```python
from build123d import *

# Parameters (mm, degrees)
BOSS_EXTRUDE1_DEPTH = 1.25
BOSS_EXTRUDE4_START = -15.5
SKETCH1_5_R         = 2
BOSS_EXTRUDE4_DEPTH = 16.75
SKETCH1_6_R         = 2
BOSS_EXTRUDE5_DEPTH = 30
CIRPATTERN1_COUNT   = 3


with BuildPart() as part:
    # Sketch1 → Boss-Extrude1 (new body, symmetric)
    with BuildSketch(Plane.XY):
        with BuildLine():
            Line((50, 2), (0, 2))
            ThreePointArc((0, 2), (1.414213562, 1.414213562), (2, 0))
            ThreePointArc((2, 0), (1.414213562, -1.414213562), (0, -2))
            Line((0, -2), (50, -2))
            ThreePointArc((50, -2), (48, 0), (50, 2))
        make_face()
    boss_extrude1 = extrude(amount=BOSS_EXTRUDE1_DEPTH, both=True)

    # Sketch1_5 → Boss-Extrude4 (add)
    with BuildSketch(Plane.XY.offset(BOSS_EXTRUDE4_START)):
        Circle(SKETCH1_5_R)
        with Locations((50, 0)):
            Circle(SKETCH1_5_R)
    boss_extrude4 = extrude(amount=BOSS_EXTRUDE4_DEPTH)

    # Sketch1_6 → Boss-Extrude5 (add)
    with BuildSketch(Plane.XY):
        Circle(SKETCH1_6_R)
    extrude(amount=BOSS_EXTRUDE5_DEPTH)

    # CirPattern1: Boss-Extrude1, Boss-Extrude4 ×3 about axis
    cirpattern1_axis = Axis((0, 0, 0), (0, 0, 1))
    for i in range(1, CIRPATTERN1_COUNT):
        add(boss_extrude1.rotate(cirpattern1_axis, i * 360 / CIRPATTERN1_COUNT))
        add(boss_extrude4.rotate(cirpattern1_axis, i * 360 / CIRPATTERN1_COUNT))


solid = part.part
```
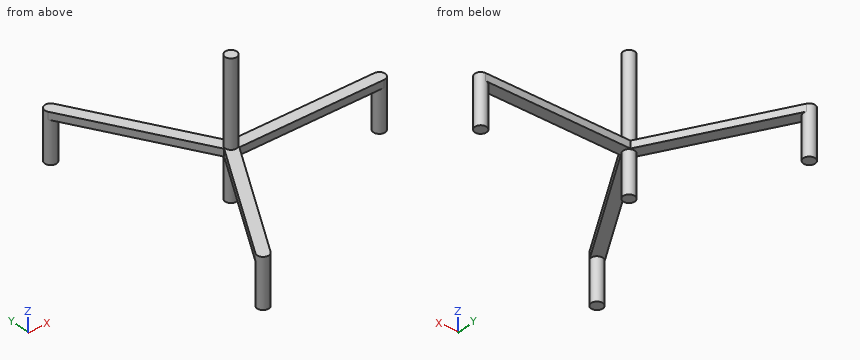
Part model, mm, in its own coordinate system. Round coordinates to 2 decimals unless told otherwise and drop trailing zeros. Order: outer loops, then holes, each group sorted by start corner. A loop starts at its lowest first (then second) coordinate and runs counter-clockwise, first axis right, second up. Notation, with made-up numbers: M -40,75 L -14,75 A31 cw -14,101 Z; hole C -1,23 d9. An arc over 180 degrees is marked long. Put each result on its own line as item: value. Start each with the question number.
1. Drill centre lines: probe 1 along Z at (x, y) = (-23.5, -37); probe 2 along Y at (x, z) = (8.5, -1); probe 3 along Y at (x, z) = (-1, 16). Where is each one in solid material? Low to high. Write a range as [from, to].
2. Drop flat-ended pins along their axis: pin 1 (12 mm diameter, centred on y = -15.5, z = 0, fed in from -X); pin 2 (3 mm diameter, centred on y = -3, z = 23, fed in from -X); pin 3 (3 mm diameter, centred on x = 26, z = 0, fed in from -Y). Give the stop position or say it passes through.
3. Slice it at C-C on z = -3. List the corners of the cut face in (x, y).
4. Slice it at A-A on z = 5.5. List the corners of the cut face in (x, y).
5. Slice it at D-D on y = -4. List the corners of the cut face in (x, z).
6. Slice it at B-B on x = 15. List the corners of the cut face in (y, z).
Findings:
1. probe 1: [-1.25, 1.25]
1. probe 2: [-2, 2]
1. probe 3: [-1.73, 1.73]
2. pin 1: x = -14.72
2. pin 2: x = -1.32
2. pin 3: y = -2
3. outline: C -25,-43.3 d4; C -25,43.3 d4; C 0,0 d4; C 50,0 d4
4. outline: C 0,0 d4
5. outline: M -4.62,-1.25 L 0,-1.25 L 0,1.25 L -4.62,1.25 Z
6. outline: M -2,-1.25 L 2,-1.25 L 2,1.25 L -2,1.25 Z
